from build123d import *

# Parameters (mm, degrees)
SALIENTE_EXTRUIR1_DEPTH = 30
CROQUIS3_W              = 4.89350096
CROQUIS3_H              = 4.01782184
SALIENTE_EXTRUIR2_DEPTH = 3
SALIENTE_EXTRUIR3_DEPTH = 21.5
REDONDEO2_R             = 3


with BuildPart() as part:
    # Croquis1 → Saliente-Extruir1 (new body)
    with BuildSketch(Plane(origin=(0, 0, 0), x_dir=(1, 0, 0), z_dir=(0, 1, 0))):
        with BuildLine():
            Line((-6, 8), (6, 8))
            ThreePointArc((6, 8), (10.242640687, 6.242640687), (12, 2))
            Line((12, 2), (12, -2))
            ThreePointArc((12, -2), (10.242640687, -6.242640687), (6, -8))
            Line((6, -8), (-6, -8))
            ThreePointArc((-6, -8), (-10.242640687, -6.242640687), (-12, -2))
            Line((-12, -2), (-12, 2))
            ThreePointArc((-12, 2), (-10.242640687, 6.242640687), (-6, 8))
        make_face()
        with BuildLine():
            Line((-6, -5), (6, -5))
            ThreePointArc((6, -5), (8.121320344, -4.121320344), (9, -2))
            Line((9, -2), (9, 2))
            ThreePointArc((9, 2), (8.121320344, 4.121320344), (6, 5))
            Line((6, 5), (-6, 5))
            ThreePointArc((-6, 5), (-8.121320344, 4.121320344), (-9, 2))
            Line((-9, 2), (-9, -2))
            ThreePointArc((-9, -2), (-8.121320344, -4.121320344), (-6, -5))
        make_face(mode=Mode.SUBTRACT)
    extrude(amount=SALIENTE_EXTRUIR1_DEPTH)

    # Croquis3 → Saliente-Extruir2 (add)
    with BuildSketch(Plane(origin=(0, 0, -8), x_dir=(-1, 0, 0), z_dir=(0, 0, -1))):
        with Locations((0, 15)):
            Rectangle(CROQUIS3_W, CROQUIS3_H)
    extrude(amount=SALIENTE_EXTRUIR2_DEPTH)

    # Croquis7 → Saliente-Extruir3 (add, symmetric)
    with BuildSketch(Plane(origin=(0, 17.00891092, 0), x_dir=(1, 0, 0), z_dir=(0, 1, 0))):
        Polygon((-2.44675048, 11), (2.44675048, 11), (25.428083774, 30.283628291), (33.597669299, 42.86368681), (31.920328163, 43.95296488), (23.913536336, 31.623586673), (1.718810011, 13), (-1.718810011, 13), (-23.913536336, 31.623586673), (-31.920328163, 43.95296488), (-33.597669299, 42.86368681), (-25.428083774, 30.283628291), align=None)
    extrude(amount=SALIENTE_EXTRUIR3_DEPTH, both=True)

    # Redondeo2
    # the kernel refuses this fillet: 3 mm, written as the material it adds along each edge
    with BuildSketch(Plane(origin=(-23.913536336, -4.49108908, -31.623586673), x_dir=(0.7660444431189832, 0, 0.6427876096865331), z_dir=(0, 1, 0)), Plane(origin=(23.913536336, -4.49108908, -31.623586673), x_dir=(0.5446390350150309, 0, -0.8386705679454215), z_dir=(0, 1, 0))) as redondeo2_piece_1:
        with BuildLine():
            CenterArc((REDONDEO2_R * 0.149451001349, REDONDEO2_R), REDONDEO2_R, 253, 17)
            Line((-REDONDEO2_R * 0.142920703374, REDONDEO2_R * 0.043695244037), (0, 0))
            Line((0, 0), (REDONDEO2_R * 0.149451001349, 0))
        make_face()
    extrude(amount=43)
    with BuildSketch(Plane(origin=(1.718810011, -4.49108908, -13), x_dir=(0.7660444431189833, 0, -0.6427876096865328), z_dir=(0, 1, 0)), Plane(origin=(-1.718810011, -4.49108908, -13), x_dir=(1, 0, 0), z_dir=(0, 1, 0))) as redondeo2_piece_2:
        with BuildLine():
            CenterArc((REDONDEO2_R * 0.363970234266, REDONDEO2_R), REDONDEO2_R, 230, 40)
            Line((-REDONDEO2_R * 0.27881737542, REDONDEO2_R * 0.233955556881), (0, 0))
            Line((0, 0), (REDONDEO2_R * 0.363970234266, 0))
        make_face()
    extrude(amount=43)
    # the kernel refuses this fillet: 3 mm, written as the material it takes off along each edge
    with BuildSketch(Plane(origin=(31.920328163, -11.562156891, -43.95296488), x_dir=(0.8386705679454225, 0, 0.5446390350150296), z_dir=(0, 1, 0))) as redondeo2_2_piece_1:
        with BuildLine():
            CenterArc((3, -2.828427125), REDONDEO2_R, 109.471220634, 70.528779366)
            Line((0, -2.828427125), (0, 0))
            Line((0, 0), (2, 0))
        make_face()
    extrude(amount=57.142135624, mode=Mode.SUBTRACT)
    with BuildSketch(Plane(origin=(-31.920328163, -11.562156891, -43.95296488), x_dir=(0.5446390350150306, 0, 0.8386705679454217), z_dir=(0, 1, 0))) as redondeo2_2_piece_2:
        with BuildLine():
            CenterArc((2.828427125, -3), REDONDEO2_R, 90, 70.528779366)
            Line((0, -2), (0, 0))
            Line((0, 0), (2.828427125, 0))
        make_face()
    extrude(amount=57.142135624, mode=Mode.SUBTRACT)


solid = part.part
Can you work these out from the model? Positions are in its coordinate system, mm. A direction names the side the tool comes from. Round coordinates to 2 decimals unless told otherwise and drop trailing zeros. Order: outer loops, then holes, each group sorted by start corner. A loop starts at its lowest first (then second) coordinate and runs counter-clockwise, first axis right, second up. Notation, with made-up numbers: (-7.5, 87.5) -> (31.5, 87.5) arc R16 ccw to (31.5, 92.5) -> close; hole circle Ø9 at (17, -7). An arc over 180 degrees is marked (long way). Write each question's results on one line, items separated by ' | '. Start each with the question number.
Item 1: If we section it at C-C, the plane z = -26: Write out the boundary of the cut face in (x, y).
Item 2: Please list where these lines run through material, in increasing order: L1, parallel to Z at x = 8, y = 16; L2, parallel to Y at x = -10.5, z = -3.5; L3, parallel to Z at x = 5, y = 26.
Item 3: Will these pins go through, and if not, where does the flat tip stop? pin 1 (12 mm diameter, centred on y = 2, z = -36.5, fed in from -X); pin 2 (3 mm diameter, centred on y = 16.5, z = 0, fed in from -X); pin 3 (1.4 mm diameter, centred on x = 0, y = 25, fed in from -Z).
Item 4: If we section it at B-B, the plane x = -3.5: Write out the boundary of the cut face in (y, z), then the cut area to 3 significant figures.
Item 5: If we section it at A-A, the plane y = 22.5: State how many separate pieces and enclosed holes the cut face has, then the cut area to 3 significant figures.
Item 6: Which directions (+Z, -Z, +X, -X, +Y, -Y) give clear straight access to the entire face, cutting with the end or side of a thin tool? Please do faces 5 (the cylindrical face through (-8.14, 14.79, 4.1)), 6 (the flat face through (13.78, 17.31, -20.51)), 7 (the flat face through (-9.1, 38.509, -18.7)), 8 (the flat face through (0.2, 30, -5.4)), 9 (the cylindrical face through (-1.7, 16.7, -13.2)).
Item 7: Thinking about a two-plate mould opening in X: for faces 1 (the flat face through (27.312, 17.31, -36.857)), 2 (the cylindrical face through (10.289, 14.79, 6.196)), 3 (the flat face through (-12, 15, 0)), 4 (the cylindrical face through (31.809, 16.708, -42.743)), which applies, +X half, -X half, draft (parallel to the pull), parting line (faces both ways), or undercut?
Results:
1) outline: (-20.32, -4.49) -> (-17.21, -4.49) -> (-17.21, 38.51) -> (-20.32, 38.51) -> close; (17.21, -4.49) -> (20.32, -4.49) -> (20.32, 38.51) -> (17.21, 38.51) -> close
2) L1: z = -18.27 to -15.66, -7.66 to -4.24, 4.24 to 7.66 | L2: y = 0 to 30 | L3: z = -15.75 to -13.14, -8 to -5, 5 to 8
3) pin 1: stops at x = -33.36 | pin 2: stops at x = -12 | pin 3: stops at z = -13
4) outline: (-4.49, -14.49) -> (38.51, -14.49) -> (38.51, -11.88) -> (-4.49, -11.88) -> close; (0, -8) -> (30, -8) -> (30, -5) -> (0, -5) -> close; (0, 5) -> (30, 5) -> (30, 8) -> (0, 8) -> close | area: 292 mm2
5) separate pieces: 2 | enclosed holes: 1 | area: 364 mm2
6) face 5: +Y, -Y | face 6: +X, +Y, -Y | face 7: +Z, -Z, +X, -X, +Y | face 8: +Z, +X, -X, +Y | face 9: -Z, +Y, -Y
7) face 1: undercut | face 2: +X half | face 3: -X half | face 4: undercut
